Part model, mm, in its own coordinate system. Face numbers are marked on the shaded views. A direction names the side the tool comes from. Coordinates: 2 decimals unless noted, no trailing zeros. Loops run counter-clockwise (first coordinate to the right, second up) from the corner with the lowest first, then second, coordinate; pieces in that order, holes last. Notation, with made-up numbers: M 69.5,86 L 124.5,86 A33 ccw 124.5,115 Z; hole C -28,10 d9. An arc over 180 degrees is marked long. Answer as a JSON object with one key per item and string values. Group by question number.
1. Saw through at C-C on x = -16. Write the cut outline in (y, z) (1 decimal).
2. Saw through at B-B on x = 0. Count the separate pieces of the cut face and the enclosed holes in it, then the cut area to 3 significant figures.
3. Drop flat-ended pins along their axis: pin 1 Ø11 at (x, z) = (40.96, -44.65) entering from -Y (3 decimals); pin 2 Ø12 at (y, z) = (-8.5, 52.5) entering from +X; pin 3 Ø5 at (x, y) = (2.5, -21) entering from -Z. Give the stop position or say it passes through.
4. Saw through at D-D on x = 51.5. Write the cut outline in (y, z) (3 decimals).
5. Drill centre lines: L1, parallel to Z at x = 0, y = -17.75; L2, parallel to X at y = -14.5, z = 5.5; L3, parallel to Z at x = 28, y = -20.75. Where is each one in solid material? Low to high.
6. Mould opens along X. For the marked faces 1, 2 and 3 say: released by +X, released by -X, zero draft, split by the parting line, or undercut.
7. 3-axis set-ups, long thin cutter, end or side, ignore diameter. For the marked faces 4 and 5: which of +Z, -Z, +X, -X, +Y, -Y reach the whole face in a straight line?
from build123d import *

# Parameters (mm, degrees)
F0_R     = 44.45
F0_R_2   = 31.75
F1_DEPTH = 25.4
F0_R_3   = 4.7625
F2_DEPTH = 9.525


with BuildPart() as f1:
    # F0 (on Front) → F1 (new body)
    with BuildSketch(Plane.XZ):
        Circle(F0_R)
        Circle(F0_R_2, mode=Mode.SUBTRACT)
    extrude(amount=F1_DEPTH)

    # F0 (on Front) → F2 (join)
    with BuildSketch(Plane.XZ):
        with BuildLine():
            ThreePointArc((30.748129, -52.209978), (49.540006, -54.013248), (49.363954, -35.135869))
            ThreePointArc((49.363954, -35.135869), (56.466669, 21.973723), (12.630065, 59.260532))
            ThreePointArc((12.630065, 59.260532), (0, 73.291495), (-12.630065, 59.260532))
            ThreePointArc((-12.630065, 59.260532), (-56.466669, 21.973723), (-49.363954, -35.135869))
            ThreePointArc((-49.363954, -35.135869), (-49.540006, -54.013248), (-30.748129, -52.209978))
            ThreePointArc((-30.748129, -52.209978), (0, -60.591495), (30.748129, -52.209978))
        make_face()
        with Locations((-40.95568, -44.653796)):
            Circle(F0_R_3, mode=Mode.SUBTRACT)
        Circle(F0_R, mode=Mode.SUBTRACT)
        with Locations((40.95568, -44.653796)):
            Circle(F0_R_3, mode=Mode.SUBTRACT)
        with Locations((0, 60.591495)):
            Circle(F0_R_3, mode=Mode.SUBTRACT)
    extrude(amount=F2_DEPTH)


solid = f1.part
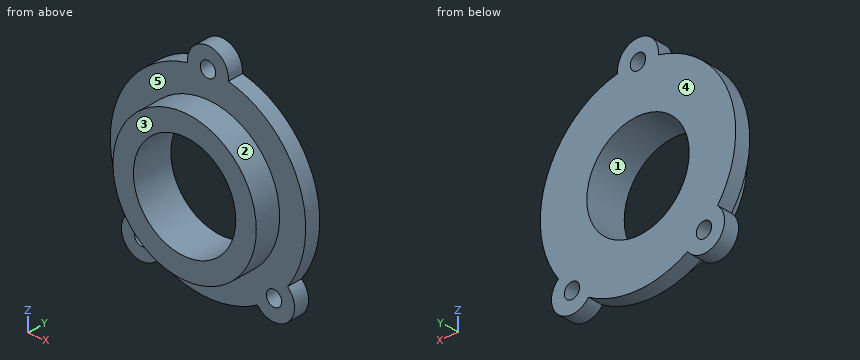
Outcome:
{
 "1": {"outline": "M -25.4,-41.5 L -9.5,-41.5 L -9.5,-58.4 L 0,-58.4 L 0,-27.4 L -25.4,-27.4 Z; M -25.4,27.4 L 0,27.4 L 0,58.4 L -9.5,58.4 L -9.5,41.5 L -25.4,41.5 Z"},
 "2": {"separate pieces": "3", "enclosed holes": "0", "area": "983 mm²"},
 "3": {"pin 1": "stops at y = -9.525", "pin 2": "stops at x = 38.85", "pin 3": "stops at z = -44.45"},
 "4": {"outline": "M -9.525,-51.732 L 0,-51.732 L 0,-37.575 L -9.525,-37.575 Z; M -9.525,-31.923 L 0,-31.923 L 0,31.923 L -9.525,31.923 Z"},
 "5": {"L1": "z = -44.45 to -31.75, 31.75 to 44.45", "L2": "x = -44.11 to -31.27, 31.27 to 44.11", "L3": "z = -34.52 to -14.97, 14.97 to 34.52"},
 "6": {"face 1": "undercut", "face 2": "split by the parting line", "face 3": "zero draft"},
 "7": {"face 4": "+Z, -Z, +X, -X, +Y", "face 5": "-Y"}
}
